Build history of the part. All positions in model axes, mm. Face numbers are marked on the shaded views. A direction names the side the tool comes from. Give positions to 0.01 mm unless a question says otherwise; leave off trailing zeros. Order: outer loops, then holes, each group sorted by start corner. A loop starts at its lowest first (then second) coordinate and runs counter-clockwise, first axis right, second up. Notation, with made-up numbers: (22.5, -1) - (75.5, -1) arc R27 ccw to (75.5, 22) - close; hole circle Ø11 at (-29.5, 67). An arc over 180 degrees is marked (long way). Answer in a Markdown table with one row per item.
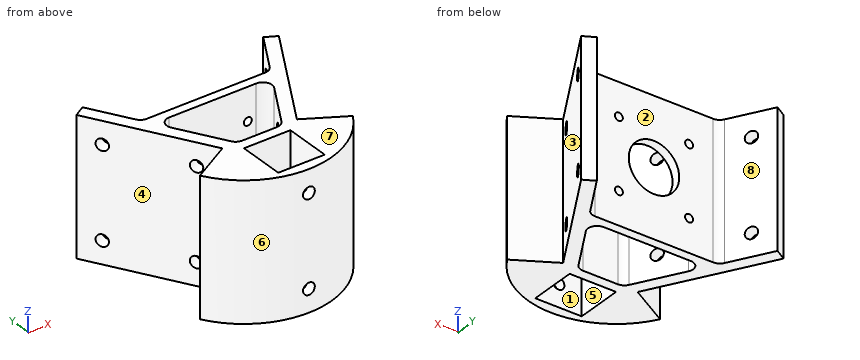
```python
from build123d import *

# Parameters (mm, degrees)
F0_W     = 20.5
F0_H     = 20.5
F1_DEPTH = 60
F2_R     = 1.75
F2_R_2   = 11.15
F3_DEPTH = 4
F4_R     = 2.6
F5_DEPTH = 5.6
F6_R     = 2.6
F7_DEPTH = 5.6
F8_R     = 2.6
F9_DEPTH = 4.501


with BuildPart() as f1:
    # F0 (on Top) → F1 (new body)
    with BuildSketch(Plane.XY):
        with BuildLine():
            Line((-16.4544826719, -9.5), (-33.7749907476, -19.5))
            ThreePointArc((-33.7749907476, -19.5), (0, -39), (33.7749907476, -19.5))
            Line((33.7749907476, -19.5), (16.4544826719, -9.5))
            Line((16.4544826719, -9.5), (44.7044826719, 39.4304353138))
            Line((44.7044826719, 39.4304353138), (39.7695460128, 42.0828742882))
            Line((39.7695460128, 42.0828742882), (29.6180688094, 24.5))
            ThreePointArc((29.6180688094, 24.5), (28.1539671943, 23.0358983849), (26.1539671943, 22.5))
            Line((26.1539671943, 22.5), (-26.1539671943, 22.5))
            ThreePointArc((-26.1539671943, 22.5), (-28.1539671943, 23.0358983849), (-29.6180688094, 24.5))
            Line((-29.6180688094, 24.5), (-39.9072594683, 42.3214009899))
            Line((-39.9072594683, 42.3214009899), (-44.7044826719, 39.4304353138))
            Line((-44.7044826719, 39.4304353138), (-16.4544826719, -9.5))
        make_face()
        with Locations((0, -24.25)):
            Rectangle(F0_W, F0_H, mode=Mode.SUBTRACT)
        with BuildLine():
            Line((-11.1428601954, -7.5), (-22.6898655792, 12.5))
            ThreePointArc((-22.6898655792, 12.5), (-22.6898655792, 16.5), (-19.225763964, 18.5))
            Line((-19.225763964, 18.5), (19.225763964, 18.5))
            ThreePointArc((19.225763964, 18.5), (22.6898655792, 16.5), (22.6898655792, 12.5))
            Line((22.6898655792, 12.5), (11.1428601954, -7.5))
            ThreePointArc((11.1428601954, -7.5), (9.6787585802, -8.9641016151), (7.6787585802, -9.5))
            Line((7.6787585802, -9.5), (-7.6787585802, -9.5))
            ThreePointArc((-7.6787585802, -9.5), (-9.6787585802, -8.9641016151), (-11.1428601954, -7.5))
        make_face(mode=Mode.SUBTRACT)
    extrude(amount=F1_DEPTH)

    # F2 (on face) → F3 (cut)
    with BuildSketch(Plane(origin=(0, 22.5, 0), x_dir=(-1, 0, 0), z_dir=(0, 1, 0))):
        with Locations((-15.5, 14.5)):
            Circle(F2_R)
        with Locations((-15.5, 45.5)):
            Circle(F2_R)
        with Locations((15.5, 45.5)):
            Circle(F2_R)
        with Locations((15.5, 14.5)):
            Circle(F2_R)
        with Locations((0, 30)):
            Circle(F2_R_2)
    extrude(amount=-F3_DEPTH, mode=Mode.SUBTRACT)

    # F4 (on face) → F5 (cut)
    with BuildSketch(Plane(origin=(-16.4544826719, -9.5, 0), x_dir=(0.5, -0.8660254038, 0), z_dir=(-0.8660254038, -0.5, 0))):
        with Locations((-46.5, 50)):
            Circle(F4_R)
        with Locations((-10, 50)):
            Circle(F4_R)
        with Locations((-10, 10)):
            Circle(F4_R)
        with Locations((-46.5, 10)):
            Circle(F4_R)
    extrude(amount=-F5_DEPTH, mode=Mode.SUBTRACT)

    # F6 (on face) → F7 (cut)
    with BuildSketch(Plane(origin=(16.4544826719, -9.5, 0), x_dir=(0.5, 0.8660254038, 0), z_dir=(0.8660254038, -0.5, 0))):
        with Locations((46.5, 50)):
            Circle(F6_R)
        with Locations((46.5, 10)):
            Circle(F6_R)
        with Locations((10, 10)):
            Circle(F6_R)
        with Locations((10, 50)):
            Circle(F6_R)
    extrude(amount=-F7_DEPTH, mode=Mode.SUBTRACT)

    # F8 (on face) → F9 (cut, through all)
    with BuildSketch(Plane(origin=(0, -34.5, 0), x_dir=(-1, 0, 0), z_dir=(0, 1, 0))):
        with Locations((0, 50)):
            Circle(F8_R)
        with Locations((0, 10)):
            Circle(F8_R)
    extrude(amount=-F9_DEPTH, mode=Mode.SUBTRACT)


solid = f1.part
```
1. Two-plate mould, pull along Y, no slides. Class the marked faces 5, 6, 7 and 8: +Y half, -Y half, draft (parallel to the pull), parting line (faces both ways), or undercut.
Check result:
| item | result |
|---|---|
| face 5 | undercut |
| face 6 | -Y half |
| face 7 | draft |
| face 8 | +Y half |
2. Cut at B-B on x = -25. Write the cut outline in (y, z), and give its area (3 significant figures).
Check result:
| item | result |
|---|---|
| outline | (-29.93, 0) - (-14.43, 0) - (-14.43, 60) - (-29.93, 60) - close; (5.3, 0) - (22.5, 0) - (22.5, 60) - (5.3, 60) - close |
| area | 1,960 mm² |
3. Probe line 1 (Z direction, x = 15.5, y = 20.05); line 2 (Z direction, x = 0, y = -37); line 3 (Y direction, x = -21.5, z = 43.5). List the from-to ranges inside material, lowest first.
Check result:
| item | result |
|---|---|
| line 1 | z = 0 to 12.75, 16.25 to 43.75, 47.25 to 60 |
| line 2 | z = 0 to 7.4, 12.6 to 47.4, 52.6 to 60 |
| line 3 | y = -32.54 to -12.41, -0.76 to 10.44, 17.79 to 22.5 |
4. Drop flat-ended pins along their axis: P1, Ø2, axis at x = -19.5, z = 30, coming from the -Y side; P2, Ø16.5, axis at x = -0.5, z = 28, coming from the -Y side; P3, Ø1.5, axis at x = 31, y = -16.5, coming from the +Z side; P4, Ø3, axis at y = 22.5, z = 38.5, coming from the -X side. Give the stop position or say it passes through.
Check result:
| item | result |
|---|---|
| P1 | stops at y = -34.33 |
| P2 | stops at y = -39 |
| P3 | passes through |
| P4 | stops at x = -35.8 |
5. Cut at C-C on z = 30. Write the cut outline in (x, y) (3 decimals).
Check result:
| item | result |
|---|---|
| outline | (-44.704, 39.43) - (-16.454, -9.5) - (-33.775, -19.5) arc R39 ccw to (33.775, -19.5) - (16.454, -9.5) - (44.704, 39.43) - (39.77, 42.083) - (29.618, 24.5) arc R4 cw to (26.154, 22.5) - (11.15, 22.5) - (11.15, 18.5) - (19.226, 18.5) arc R4 cw to (22.69, 12.5) - (11.143, -7.5) arc R4 cw to (7.679, -9.5) - (-7.679, -9.5) arc R4 cw to (-11.143, -7.5) - (-22.69, 12.5) arc R4 cw to (-19.226, 18.5) - (-11.15, 18.5) - (-11.15, 22.5) - (-26.154, 22.5) arc R4 cw to (-29.618, 24.5) - (-39.907, 42.321) - close; hole (-10.25, -34.5) - (10.25, -34.5) - (10.25, -14) - (-10.25, -14) - close |
6. Cut at A-A on z = 45.5. Count the separate pieces of the cut face and the enclosed holes in it, and give its area (3 significant figures).
Check result:
| item | result |
|---|---|
| separate pieces | 2 |
| enclosed holes | 1 |
| area | 1,880 mm² |
7. Which spindle directions (+Z, -Z, +X, -X, +Y, -Y) get a long thin tool onto all of the face, cutting with end or side? Do the marked faces 1, 2, 3 and 4. Say none if no direction does.
Check result:
| item | result |
|---|---|
| face 1 | +Z, -Z |
| face 2 | +Z, -Z, +Y |
| face 3 | +Z, -Z, +X |
| face 4 | +Z, -Z, -X |
8. Cut at D-D on x = 5.5. Write the cut outline in (y, z), and give its area (3 significant figures).
Check result:
| item | result |
|---|---|
| outline | (-38.61, 0) - (-34.5, 0) - (-34.5, 60) - (-38.61, 60) - close; (-14, 0) - (-9.5, 0) - (-9.5, 60) - (-14, 60) - close; (18.5, 0) - (22.5, 0) - (22.5, 20.3) - (18.5, 20.3) - close; (18.5, 39.7) - (22.5, 39.7) - (22.5, 60) - (18.5, 60) - close |
| area | 679 mm² |
